```python
from build123d import *

# Parameters (mm, degrees)
BOSS_EXTRUDE1_DEPTH      = 19.05
SKETCH3_R                = 31.75
BOSS_EXTRUDE2_DEPTH      = 41.402
BOSS_EXTRUDE2_DEPTH_BACK = 60.198


with BuildPart() as part:
    # Sketch1 → Boss-Extrude1 (new body)
    with BuildSketch(Plane(origin=(0, 0, 0), x_dir=(1, 0, 0), z_dir=(0, 1, 0))):
        with BuildLine():
            Line((-49.276, 31.75), (49.276, 31.75))
            ThreePointArc((49.276, 31.75), (81.026, 0), (49.276, -31.75))
            Line((49.276, -31.75), (-49.276, -31.75))
            ThreePointArc((-49.276, -31.75), (-81.026, 0), (-49.276, 31.75))
        make_face()
    extrude(amount=BOSS_EXTRUDE1_DEPTH)

    # Sketch3 → Boss-Extrude2 (add, two sides)
    with BuildSketch(Plane(origin=(0, 19.05, 0), x_dir=(1, 0, 0), z_dir=(0, 1, 0))) as boss_extrude2_sk:
        with Locations(Location((-49.276, 0, 0), (0, 0, 270))):  # turned: the seam where the file's is
            Circle(SKETCH3_R)
    extrude(amount=BOSS_EXTRUDE2_DEPTH)
    extrude(boss_extrude2_sk.sketch, amount=-BOSS_EXTRUDE2_DEPTH_BACK)


solid = part.part
```
CAD build for the part. Positions are in the model's coordinates, mm. A direction names the side the tool comes from. Round coordinates to 2 decimals unless told otherwise and drop trailing zeros. Write each loop counter-clockwise with the first axis right and the second up, starting at its lowest first coordinate (ties: lowest second). Pieces come first, ordered by that corner, then holes. Notation, with made-up numbers: (31.5, 50.5) -> (83.5, 50.5) arc R31 ccw to (83.5, 78.5) -> close; hole circle Ø1 at (-23, 9.5). An arc over 180 degrees is marked (long way). Answer in a Markdown table with one row per item. Add a question column.
Item 1: Drill centre lines: line 1 (Y direction, x = 11.5, z = 8); line 2 (X direction, y = 49, z = 6); line 3 (X direction, y = 33, z = -12). Where is each one in solid material? Low to high. Write a range as from..to.
Item 2: Drop flat-ended pins along their axis: pin 1 Ø10 at (x, y) = (-42.5, 39) entering from +Z; pin 2 Ø1 at (x, z) = (38.5, -22.5) entering from +Y; pin 3 Ø1.5 at (x, z) = (64, 4.5) entering from -Y. Give the stop position or say it passes through.
Item 3: Saw through at D-D, the plane y = -27. Write the cut outline in (x, z).
Item 4: Saw through at C-C, the plane y = 16. Write the cut outline in (x, z), then the cut area to 4 significant figures.
Item 5: Which spindle directions (+Z, -Z, +X, -X, +Y, -Y) get a long thin tool onto all of the face, cutting with end or side? Do faces 1 (the face through (-77.444, 8.941, 14.651)), 2 (the face through (-49, 60.452, 0)). Say none if no direction does.
Item 6: Mould opens along Z. For faces 3 (the face through (81.02, 9.39, -0.7)), 4 (the face through (-49, -41.148, 0)), 5 (the face through (1, 9, 31.75)) say: pulls with the +Z half, pulls with the -Z half, needs draft (parallel to the pull), parting line crosses it, or undercut.
Item 7: Saw through at B-B, the plane x = -6. Write the cut outline in (y, z).
Item 8: Saw through at A-A, the plane z = 0. Write the cut outline in (x, y), then the cut area to 3 significant figures.
Findings below:
| question | item | result |
|---|---|---|
| 1 | line 1 | y = 0..19.05 |
| 1 | line 2 | x = -80.45..-18.1 |
| 1 | line 3 | x = -78.67..-19.88 |
| 2 | pin 1 | stops at z = 31.7 |
| 2 | pin 2 | stops at y = 19.05 |
| 2 | pin 3 | stops at y = 0 |
| 3 | outline | circle Ø63.5 at (-49.28, 0) |
| 4 | outline | (-49.28, -31.75) -> (49.28, -31.75) arc R31.75 ccw to (49.28, 31.75) -> (-49.28, 31.75) arc R31.75 ccw to start |
| 4 | area | 9,425 mm^2 |
| 5 | face 1 | none |
| 5 | face 2 | +Z, -Z, +X, -X, +Y |
| 6 | face 3 | parting line crosses it |
| 6 | face 4 | needs draft |
| 6 | face 5 | pulls with the +Z half |
| 7 | outline | (0, -31.75) -> (19.05, -31.75) -> (19.05, 31.75) -> (0, 31.75) -> close |
| 8 | outline | (-81.03, -41.15) -> (-17.53, -41.15) -> (-17.53, 0) -> (81.03, 0) -> (81.03, 19.05) -> (-17.53, 19.05) -> (-17.53, 60.45) -> (-81.03, 60.45) -> close |
| 8 | area | 8,330 mm^2 |
